For this review, take the finished solid that the model builds, in its own axes (mm). A direction names the side the tool comes from. Coordinates: 2 decimals unless noted, no trailing zeros. Order: outer loops, then holes, each group sorted by start corner. A loop starts at its lowest first (then second) coordinate and runs counter-clockwise, first axis right, second up. Notation, with made-up numbers: (20.5, -15.75) -> (68.5, -15.75) arc R19 cw to (68.5, -0.75) -> close; hole circle Ø8 at (18.25, 48). An arc over 180 degrees is marked (long way). Answer as a JSON object with one key per item and string values. Group by question number.
1) Draft analysis for pull direction X (two halves, no side actions). For faces 1 (the flat face through (47, 10, 12)), 2 (the flat face through (49, 0, 12)), 3 (the flat face through (9.5, 8, 12)), state which applies: +X half, -X half, draft (parallel to the pull), parting line (faces both ways), or undercut.
2) Add section D-D, the plane x = 31. Write out the cut boundary in (y, z), then the cut area to 3 significant figures.
3) For pin 1 (5 mm diameter, centred on x = 14, y = 10.5, fed in from +Z); pin 2 (3 mm diameter, centred on y = 8.5, z = 12.5, fed in from +X); pin 3 (7.5 mm diameter, centred on x = 21.5, z = 11.5, fed in from -Y); pin 4 (5.5 mm diameter, centred on x = 3, z = 9.5, fed in from +Y), all flat-tipped, find the tip position at first contact; note any pin that passes through.
4) Add section A-A, the plane y = 14.75. Write out the cut boundary in (x, z), then the cut area to 3 significant figures.
5) Add section C-C, the plane x = 3.2. Write out the cut boundary in (y, z).
6) Add section B-B, the plane z = 12.5. Write out the cut boundary in (x, y), then the cut area to 3 significant figures.
7) Machinability: for faces 4 (the flat face through (5, 0, 12)), 5 (the flat face through (27, 19, 0)), 6 (the flat face through (44.5, 7, 12)), which of the approach directions +Z, -Z, +X, -X, +Y, -Y give a long, thin tool a straight path to every point of the face, cutting with its end or side? Answer none if there is none.
8) Wall thickness on L1, parallel to X at y = -1.65, z = 12.5; L2, parallel to X at y = 8.5, z = 12.25; L3, parallel to Y at x = 24, z = 17.75: over which ranges is each line inside the solid? List them lowest first.
from build123d import *

# Parameters (mm, degrees)
EXTRUDE_THIN1_DEPTH = 25
CUT_EXTRUDE1_DEPTH  = 64.618000597
SKETCH3_R           = 1.6
CUT_EXTRUDE2_DEPTH  = 63.777384463


with BuildPart() as part:
    # Sketch1 → Extrude-Thin1 (new body)
    with BuildSketch(Plane.XY):
        Polygon((0, 0), (7, 0), (7, 20), (47, 20), (47, 0), (54, 0), (54, -2.5), (44.5, -2.5), (44.5, 17.5), (9.5, 17.5), (9.5, -2.5), (0, -2.5), align=None)
    extrude(amount=EXTRUDE_THIN1_DEPTH)

    # Sketch2 → Cut-Extrude1 (cut, through all)
    with BuildSketch(Plane(origin=(0, 20, 0), x_dir=(1, 0, 0), z_dir=(0, 1, 0))):
        Polygon((0, -8), (13.856406461, 0), (7, 0), (0, 0), align=None)
        Polygon((0, -17), (13.856406461, -25), (7, -25), (0, -25), align=None)
        Polygon((54, -17), (40.143593539, -25), (47, -25), (54, -25), align=None)
        Polygon((54, -8), (40.143593539, 0), (47, 0), (54, 0), align=None)
    extrude(amount=-CUT_EXTRUDE1_DEPTH, mode=Mode.SUBTRACT)

    # Sketch3 → Cut-Extrude2 (cut, through all)
    with BuildSketch(Plane(origin=(0, 0, 0), x_dir=(1, 0, 0), z_dir=(0, 1, 0))):
        with Locations(Location((50.8, -12.5, 0), (0, 0, 270))):
            Circle(SKETCH3_R)
        with Locations(Location((3.2, -12.5, 0), (0, 0, 270))):
            Circle(SKETCH3_R)
    extrude(amount=-CUT_EXTRUDE2_DEPTH, mode=Mode.SUBTRACT)


solid = part.part
Output values:
{
 "1": {"face 1": "+X half", "face 2": "draft", "face 3": "undercut"},
 "2": {"outline": "(17.5, 0) -> (20, 0) -> (20, 25) -> (17.5, 25) -> close", "area": "62.5 mm²"},
 "3": {"pin 1": "passes through", "pin 2": "stops at x = 47", "pin 3": "stops at y = 17.5", "pin 4": "stops at y = 0"},
 "4": {"outline": "(7, 3.96) -> (9.5, 2.52) -> (9.5, 22.48) -> (7, 21.04) -> close; (44.5, 2.52) -> (47, 3.96) -> (47, 21.04) -> (44.5, 22.48) -> close", "area": "92.6 mm²"},
 "5": {"outline": "(-2.5, 6.15) -> (0, 6.15) -> (0, 10.9) -> (-2.5, 10.9) -> close; (-2.5, 14.1) -> (0, 14.1) -> (0, 18.85) -> (-2.5, 18.85) -> close"},
 "6": {"outline": "(0, -2.5) -> (1.6, -2.5) -> (1.6, 0) -> (0, 0) -> close; (4.8, -2.5) -> (9.5, -2.5) -> (9.5, 17.5) -> (44.5, 17.5) -> (44.5, -2.5) -> (49.2, -2.5) -> (49.2, 0) -> (47, 0) -> (47, 20) -> (7, 20) -> (7, 0) -> (4.8, 0) -> close; (52.4, -2.5) -> (54, -2.5) -> (54, 0) -> (52.4, 0) -> close", "area": "219 mm²"},
 "7": {"face 4": "+Z, -Z, -X, +Y", "face 5": "-Z, +X, -X, +Y, -Y", "face 6": "+Z, -Z, -Y"},
 "8": {"L1": "x = 0 to 1.6, 4.8 to 9.5, 44.5 to 49.2, 52.4 to 54", "L2": "x = 7 to 9.5, 44.5 to 47", "L3": "y = 17.5 to 20"}
}
